```python
from build123d import *

# Parameters (mm, degrees)
SKETCH_1_R               = 16.3
EXTRUDE_1_DEPTH          = 19.75
SKETCH_2_W               = 36.5
SKETCH_2_H               = 2.5
EXTRUDE_2_DEPTH          = 39.5
SKETCH_3_W               = 44.844436064
SKETCH_3_H               = 25.506740045
CUT_EXTRUDE_1_DEPTH      = 50
EXTRUDE_3_DEPTH          = 5.05
SKETCH_5_R               = 14.25
CUT_EXTRUDE_2_DEPTH      = 29.4
SKETCH_6_R               = 2.5
CUT_EXTRUDE_3_DEPTH      = 44.930797853
CUT_EXTRUDE_6_REACH      = 49.993
SKETCH_9_R               = 7.5
SKETCH_12_R              = 1.15
CUT_EXTRUDE_9_DEPTH      = 34.662664779
SKETCH_13_R              = 2
CUT_EXTRUDE_10_DEPTH     = 1
SKETCH_14_W              = 2.8
SKETCH_14_H              = 12
CUT_EXTRUDE_11_DEPTH     = 1.3
SKETCH_15_W              = 2.8
SKETCH_15_H              = 12
CUT_EXTRUDE_12_DEPTH     = 1.3
EXTRUDE_5_REACH          = 40.183
EXTRUDE_5_END_RADIUS     = 16.3
SKETCH_16_W              = 4
SKETCH_16_H              = 5
SKETCH_17_W              = 1
SKETCH_17_H              = 2
CUT_EXTRUDE_13_DEPTH     = 2.5
SKETCH_19_R              = 8.51898124
SKETCH_19_R_2            = 6.5
EXTRUDE_6_DEPTH          = 2.25
CUT_EXTRUDE_18_REACH     = 49.993
SKETCH_20_R              = 1.15
PATTERN_CIRCULAR_1_COUNT = 4
CUT_EXTRUDE_8_DEPTH      = 45.587021654
SKETCH_18_W              = 26.346157216
SKETCH_18_H              = 2.75
CUT_EXTRUDE_16_DEPTH     = 12.5
FILLET_1_R               = 2
FILLET_2_R               = 1
SKETCH_21_R              = 2.1
CUT_EXTRUDE_19_DEPTH     = 2.5


with BuildPart() as part:
    # 草图1 → 凸台-拉伸1 (new, symmetric)
    with BuildSketch(Plane(origin=(0, 0, 0), x_dir=(1, 0, 0), z_dir=(0, 1, 0))):
        with Locations(Location((0, 0, 0), (0, 0, 270))):
            Circle(SKETCH_1_R)
    extrude(amount=EXTRUDE_1_DEPTH, both=True)

    # 草图2 → 凸台-拉伸2 (add, through all)
    with BuildSketch(Plane.XZ.offset(19.75)):
        with Locations((3.6, -8.35)):
            Rectangle(SKETCH_2_W, SKETCH_2_H)
    extrude(amount=-EXTRUDE_2_DEPTH)

    # 草图3 → 切除-拉伸1 (cut)
    with BuildSketch(Plane.XZ.offset(19.75)):
        with Locations((-0.572218032, 5.653370022)):
            Rectangle(SKETCH_3_W, SKETCH_3_H)
    extrude(amount=-CUT_EXTRUDE_1_DEPTH, mode=Mode.SUBTRACT)

    # 草图4 → 凸台-拉伸3 (add)
    with BuildSketch(Plane.XZ.offset(19.75)):
        with BuildLine():
            Line((-14.65, -7.146152811), (-7.996542478, 4.549209646))
            ThreePointArc((-7.996542478, 4.549209646), (1.047927533, 9.140122969), (8.818653972, 2.621324497))
            ThreePointArc((8.818653972, 2.621324497), (13.721037439, -4.401937543), (21.85, -7.1))
            Line((21.85, -7.1), (-14.65, -7.146152811))
        make_face()
    extrude_3 = extrude(amount=-EXTRUDE_3_DEPTH)

    # 镜向1: 凸台-拉伸3 across plane
    add(extrude_3.mirror(Plane.ZX))

    # 草图5 → 切除-拉伸2 (cut)
    with BuildSketch(Plane(origin=(0, -14.7, 0), x_dir=(1, 0, 0), z_dir=(0, 1, 0))):
        Circle(SKETCH_5_R)
    extrude(amount=CUT_EXTRUDE_2_DEPTH, mode=Mode.SUBTRACT)

    # 草图6 → 切除-拉伸3 (cut, through all)
    with BuildSketch(Plane(origin=(0, -14.7, 0), x_dir=(1, 0, 0), z_dir=(0, 1, 0))):
        with Locations(Location((0, 0, 0), (0, 0, 270))):
            Circle(SKETCH_6_R)
    extrude(amount=-CUT_EXTRUDE_3_DEPTH, mode=Mode.SUBTRACT)

    # 草图9 → 切除-拉伸6 (cut, up to next)
    with BuildSketch(Plane(origin=(0, 19.75, 0), x_dir=(1, 0, 0), z_dir=(0, 1, 0)), mode=Mode.PRIVATE) as cut_extrude_6_sk1:
        with Locations(Location((0, 0, 0), (0, 0, 270))):
            Circle(SKETCH_9_R)
    cut_extrude_6_tool1 = extrude(cut_extrude_6_sk1.sketch, amount=-CUT_EXTRUDE_6_REACH, mode=Mode.PRIVATE) & part.part
    add(cut_extrude_6_tool1.solids().sort_by_distance((0, 19.75, 0))[0], mode=Mode.SUBTRACT)

    # 草图12 → 切除-拉伸9 (cut, through all)
    with BuildSketch(Plane.XY.offset(-7.1)):
        with Locations((17.5, 0)):
            Circle(SKETCH_12_R)
    extrude(amount=-CUT_EXTRUDE_9_DEPTH, mode=Mode.SUBTRACT)

    # 草图13 → 切除-拉伸10 (cut)
    with BuildSketch(Plane.XY.offset(-7.1)):
        with Locations((17.5, 0)):
            Circle(SKETCH_13_R)
    extrude(amount=-CUT_EXTRUDE_10_DEPTH, mode=Mode.SUBTRACT)

    # 草图14 → 切除-拉伸11 (cut)
    with BuildSketch(Plane.XY.offset(-7.1)):
        with Locations((21.85, 0)):
            Rectangle(SKETCH_14_W, SKETCH_14_H)
    extrude(amount=-CUT_EXTRUDE_11_DEPTH, mode=Mode.SUBTRACT)

    # 草图15 → 切除-拉伸12 (cut)
    with BuildSketch(Plane.XY.offset(-7.1)):
        with Locations((-14.672423113, 0)):
            Rectangle(SKETCH_15_W, SKETCH_15_H)
    extrude(amount=-CUT_EXTRUDE_12_DEPTH, mode=Mode.SUBTRACT)

    # 凸台-拉伸5: up to this cylinder (the profile starts outside it)
    extrude_5_end = Plane(origin=(0, 13.4, 0), z_dir=(0, -1, 0)) * Cylinder(EXTRUDE_5_END_RADIUS, 113.966, mode=Mode.PRIVATE)
    # 草图16 → 凸台-拉伸5 (add, up to the surface)
    with BuildSketch(Plane(origin=(0, 0, -15.1), x_dir=(-1, 0, 0), z_dir=(0, 0, -1)), mode=Mode.PRIVATE) as extrude_5_sk1:
        with Locations((11.65, 13.4)):
            Rectangle(SKETCH_16_W, SKETCH_16_H)
    extrude_5_tool1 = extrude(extrude_5_sk1.sketch, amount=-EXTRUDE_5_REACH, mode=Mode.PRIVATE) - extrude_5_end
    extrude_5 = extrude_5_tool1.solids().sort_by_distance((-11.65, 13.4, -15.1))[0]
    add(extrude_5)

    # 镜向4: 凸台-拉伸5 across plane
    add(extrude_5.mirror(Plane.ZX))

    # 草图17 → 切除-拉伸13 (cut)
    with BuildSketch(Plane(origin=(0, 0, -15.1), x_dir=(-1, 0, 0), z_dir=(0, 0, -1))):
        with Locations((11.65, 13.4)):
            Rectangle(SKETCH_17_W, SKETCH_17_H)
    cut_extrude_13 = extrude(amount=-CUT_EXTRUDE_13_DEPTH, mode=Mode.SUBTRACT)

    # 镜向5: 切除-拉伸13 across plane
    add(cut_extrude_13.mirror(Plane.ZX), mode=Mode.SUBTRACT)

    # 草图19 → 凸台-拉伸6 (add)
    with BuildSketch(Plane(origin=(0, 19.75, 0), x_dir=(1, 0, 0), z_dir=(0, 1, 0))):
        Circle(SKETCH_19_R)
        with Locations(Location((0, 0, 0), (0, 0, 270))):
            Circle(SKETCH_19_R_2, mode=Mode.SUBTRACT)
    extrude(amount=-EXTRUDE_6_DEPTH)

    # 草图20 → 切除-拉伸18 (cut, up to next)
    with BuildSketch(Plane.XZ.offset(19.75), mode=Mode.PRIVATE) as cut_extrude_18_sk1:
        with Locations(Location((0, 6, 0), (0, 0, 270))):
            Circle(SKETCH_20_R)
    cut_extrude_18_tool1 = extrude(cut_extrude_18_sk1.sketch, amount=-CUT_EXTRUDE_18_REACH, mode=Mode.PRIVATE) & part.part
    cut_extrude_18 = cut_extrude_18_tool1.solids().sort_by_distance((0, -19.75, 6))[0]
    add(cut_extrude_18, mode=Mode.SUBTRACT)

    # 阵列(圆周)1: 切除-拉伸18 ×4 about axis
    pattern_circular_1_axis = Axis((0, 0, 0), (0, 1, 0))
    for i in range(1, PATTERN_CIRCULAR_1_COUNT):
        add(cut_extrude_18.rotate(pattern_circular_1_axis, i * 360 / PATTERN_CIRCULAR_1_COUNT), mode=Mode.SUBTRACT)

    # 草图7 → 切除-拉伸8 (cut, through all)
    with BuildSketch(Plane.ZY.offset(14.65)):
        Polygon((-7.1, 19.75), (9.2, 18.323934785), (9.2, 19.75), align=None)
    cut_extrude_8 = extrude(amount=-CUT_EXTRUDE_8_DEPTH, mode=Mode.SUBTRACT)

    # 镜向3: 切除-拉伸8 across plane
    add(cut_extrude_8.mirror(Plane.ZX), mode=Mode.SUBTRACT)

    # 草图18 → 切除-拉伸16 (cut)
    with BuildSketch(Plane(origin=(0, 0, -9.6), x_dir=(-1, 0, 0), z_dir=(0, 0, -1))):
        with Locations((0, 18.375)):
            Rectangle(SKETCH_18_W, SKETCH_18_H)
    cut_extrude_16 = extrude(amount=CUT_EXTRUDE_16_DEPTH, mode=Mode.SUBTRACT)

    # 镜向6: 切除-拉伸16 across plane
    add(cut_extrude_16.mirror(Plane.ZX), mode=Mode.SUBTRACT)

    # 圆角1
    fillet_1_edges = [part.edges().sort_by_distance(p)[0] for p in [
        (12.355262037, 0, -7.1),
    ]]
    fillet(fillet_1_edges, radius=FILLET_1_R)

    # 圆角2
    fillet_2_edges = [part.edges().sort_by_distance(p)[0] for p in [
        (-12.355262037, 0, -7.1),
    ]]
    fillet(fillet_2_edges, radius=FILLET_2_R)

    # 草图21 → 切除-拉伸19 (cut)
    with BuildSketch(Plane.XZ.offset(19.75)):
        with Locations(Location((0, 6, 0), (0, 0, 270))):
            Circle(SKETCH_21_R)
        with Locations(Location((-6, 0, 0), (0, 0, 270))):
            Circle(SKETCH_21_R)
        with Locations(Location((6, 0, 0), (0, 0, 270))):
            Circle(SKETCH_21_R)
        with Locations(Location((0, -6, 0), (0, 0, 270))):
            Circle(SKETCH_21_R)
    extrude(amount=-CUT_EXTRUDE_19_DEPTH, mode=Mode.SUBTRACT)


solid = part.part
```
The model under review builds one solid part; all positions refer to its coordinate system, in mm. A direction names the side the tool comes from. Round coordinates to 2 decimals unless told otherwise and drop trailing zeros. Loops run counter-clockwise (first coordinate to the right, second up) from the corner with the lowest first, then second, coordinate; pieces in that order, holes last. Notation, with made-up numbers: (-37.75, 89) - (5.25, 89) arc R29 ccw to (5.25, 120) - close; hole circle Ø11 at (9.25, -24). An arc over 180 degrees is marked (long way). Use a Markdown table: item, result. Add a question column.
Q1. Add section B-B (x = -6). State how many separate pieces and enclosed holes the cut face has, plus the area to 3 significant figures.
Q2. For probe 1 along Z at (x, y) = (0, -18.1); probe 2 along Z at (x, y) = (0, -18.5); probe 3 along Y at (x, z) = (-6, -11.25), list the stretches that pass through material, from the lowest coordinate up.
Q3. Insertion check: pin 1 Ø2 at (x, y) = (-12.5, -14.5) entering from -Z; pin 2 Ø10 at (x, y) = (17.5, -2) entering from -Z; pin 3 Ø1.4 at (x, y) = (17.5, 0) entering from +Z; pin 4 Ø10 at (x, y) = (15, 15) entering from -Z. Each pin has a flat end and moves straight along its axis. Give the tip position at first contact, or say it passes through.
Q4. Machinability: for faces 4 (the face through (-12, 13, -12.6)), 5 (the face through (15.9, -1.2, -7.6)), 6 (the face through (-7.15, -15.99, 0.05)), 7 (the face through (21, 0, -8.4)), which of the approach directions +Z, -Z, +X, -X, +Y, -Y give a long, thin tool a straight path to every point of the face, cutting with its end or side? Answer none if there is none.
Q5. Add section D-D (y = -7.5). State the section outline as (x, z) points.
Q6. Add section A-A (y = 0). State the section outline as (x, z) points, plus the area to 3 significant figures.
Q7. The part is to be moulded in two halves that separate along Y. For faces 1 (the face through (0.826, 19.727, -6.836)), 2 (the face through (3, -19.75, -8)), 3 (the face through (-14, -6, -8)), say which applies: pulls with the +Y half, pulls with the -Y half, needs draft (parallel to the pull), parting line crosses it, or undercut.
Q8. Add section C-C (z = 6). State the section outline as (x, y) points, plus the area to 3 significant figures.
Worked answers:
| question | item | result |
|---|---|---|
| 1 | separate pieces | 3 |
| 1 | enclosed holes | 0 |
| 1 | area | 194 mm² |
| 2 | probe 1 | -9.6 to -8.1, -3.9 to -2.5, 2.5 to 3.9, 8.1 to 9.2 |
| 2 | probe 2 | -9.6 to -8.1, -3.9 to -2.5, 2.5 to 3.9 |
| 2 | probe 3 | -17 to -14.7, 14.7 to 17 |
| 3 | pin 1 | z = -15.1 |
| 3 | pin 2 | z = -10.46 |
| 3 | pin 3 | through |
| 3 | pin 4 | z = -12.87 |
| 4 | face 4 | -Z |
| 4 | face 5 | +Z |
| 4 | face 6 | -Y |
| 4 | face 7 | +Z, +X |
| 5 | outline | (-14.67, -7.1) arc R16.3 ccw to (-14.65, -7.15) - (-14.65, -9.6) - (-13.17, -9.6) arc R16.3 ccw to (13.17, -9.6) - (21.85, -9.6) - (21.85, -7.1) - (13.46, -7.1) arc R2 ccw to (11.81, -7.98) arc R14.25 cw to (-12.07, -7.57) arc R1 ccw to (-12.92, -7.1) - close |
| 6 | outline | (-14.65, -9.6) - (-13.17, -9.6) arc R16.3 ccw to (13.17, -9.6) - (16.35, -9.6) - (16.35, -8.1) - (15.5, -8.1) - (15.5, -7.1) - (13.46, -7.1) arc R2 ccw to (11.81, -7.98) arc R14.25 cw to (-12.07, -7.57) arc R1 ccw to (-12.92, -7.1) - (-13.27, -7.1) - (-13.27, -8.4) - (-14.65, -8.4) - close; (18.65, -9.6) - (21.85, -9.6) - (21.85, -8.4) - (20.45, -8.4) - (20.45, -7.1) - (19.5, -7.1) - (19.5, -8.1) - (18.65, -8.1) - close |
| 6 | area | 78.2 mm² |
| 7 | face 1 | pulls with the +Y half |
| 7 | face 2 | pulls with the -Y half |
| 7 | face 3 | undercut |
| 8 | outline | (-6.97, -18.6) - (-2.1, -18.6) - (-2.1, -17.25) - (-1.15, -17.25) - (-1.15, -14.7) - (-6.97, -14.7) - close; (-6.97, 14.7) - (-4.5, 14.7) - (-4.5, 17.5) - (-2.5, 17.5) - (-2.5, 18.6) - (-6.97, 18.6) - close; (1.15, -17.25) - (2.1, -17.25) - (2.1, -18.6) - (6.97, -18.6) - (6.97, -14.7) - (1.15, -14.7) - close; (2.5, 17.5) - (4.5, 17.5) - (4.5, 14.7) - (6.97, 14.7) - (6.97, 18.6) - (2.5, 18.6) - close |
| 8 | area | 66.6 mm² |
